The model under review builds one solid part; all positions refer to its coordinate system, in mm. Face numbers are marked on the shaded views. A direction names the side the tool comes from. Coordinates: 2 decimals unless noted, no trailing zeros. Order: outer loops, then holes, each group sorted by start corner. A loop starts at its lowest first (then second) coordinate and runs counter-clockwise, first axis right, second up.
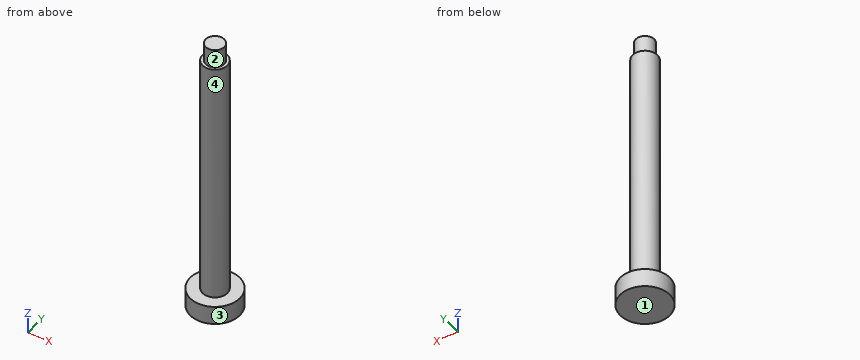
from build123d import *

# Parameters (mm, degrees)
SKETCH1_R           = 2
BOSS_EXTRUDE1_DEPTH = 40
SKETCH3_R           = 1.5
BOSS_EXTRUDE2_DEPTH = 43
SKETCH4_R           = 4
BOSS_EXTRUDE3_DEPTH = 3


with BuildPart() as part:
    # Sketch1 → Boss-Extrude1 (new body)
    with BuildSketch(Plane.XY):
        Circle(SKETCH1_R)
    extrude(amount=BOSS_EXTRUDE1_DEPTH)

    # Sketch3 → Boss-Extrude2 (add)
    with BuildSketch(Plane.XY):
        Circle(SKETCH3_R)
    extrude(amount=BOSS_EXTRUDE2_DEPTH)

    # Sketch4 → Boss-Extrude3 (add)
    with BuildSketch(Plane.XY):
        Circle(SKETCH4_R)
    extrude(amount=-BOSS_EXTRUDE3_DEPTH)


solid = part.part
(1) Insertion check: pin 1 Ø4 at (y, z) = (0, 31) entering from -X; pin 2 Ø4 at (y, z) = (-2.5, 7) entering from -X; pin 3 Ø3 at (x, z) = (2.5, 12) entering from +Y. Each pin has a flat end and moves straight along its axis. Give the tip position at first contact, or say it passes through.
(2) The part is to be moulded in two halves that separate along X. For the marked faces 1 and 2, say which applies: +X half, -X half, draft (parallel to the pull), parting line (faces both ways), or undercut.
(3) Consider section C-C (z = 39.5). Give the boundary of the cut face in (x, y).
(4) Tool access review of the marked faces 3 and 4: name each direction out of +Z, -Z, +X, -X, +Y, -Y from which nothing blocks a thin tool from reaching the whole face with its end or side.
(5) Consider section D-D (y = 2.5). Give the boundary of the cut face in (x, z).
(6) Consider section A-A (x = 0). Give the boundary of the cut face in (y, z), then the cut area to 3 significant figures.
(7) Wall thickness on line 1 (Z direction, x = 0.5, y = -3); line 2 (Z direction, x = -1.75, y = 0.5); line 3 (X direction, y = -0.75, z = 6): over which ranges is each line inside the solid? List them lowest first.
Findings:
1. pin 1: stops at x = -2
1. pin 2: stops at x = -1.94
1. pin 3: stops at y = 1.73
2. face 1: draft
2. face 2: parting line
3. outline: circle Ø4 at (0, 0)
4. face 3: +Z, -Z
4. face 4: +Z
5. outline: (-3.12, -3) - (3.12, -3) - (3.12, 0) - (-3.12, 0) - close
6. outline: (-4, -3) - (4, -3) - (4, 0) - (2, 0) - (2, 40) - (1.5, 40) - (1.5, 43) - (-1.5, 43) - (-1.5, 40) - (-2, 40) - (-2, 0) - (-4, 0) - close
6. area: 193 mm2
7. line 1: z = -3 to 0
7. line 2: z = -3 to 40
7. line 3: x = -1.85 to 1.85
